```python
from build123d import *

# Parameters (mm, degrees)
F0_R     = 4.7625
F1_DEPTH = 19.05
F4_R     = 6.0191962191


with BuildPart() as f1:
    # F0 (on Top) → F1 (new body)
    with BuildSketch(Plane.XY):
        Polygon((5.2232627241, 4.1654130256), (0, 6.6808037809), (-5.2232627241, 4.1654130256), (-6.5133020818, -1.4866186969), (-2.8986921248, -6.0191962191), (2.8986921248, -6.0191962191), (6.5133020818, -1.4866186969), align=None)
        Circle(F0_R, mode=Mode.SUBTRACT)
        Circle(F0_R)
    extrude(amount=F1_DEPTH)

    # F2 (on face) → F5 section 0
    with BuildSketch(Plane.XY.offset(19.05)):
        with BuildLine():
            ThreePointArc((4.7059970769, -3.7529074911), (5.6814189661, -1.9880145009), (6.0191962191, 0))
            ThreePointArc((6.0191962191, 0), (5.9813487804, 0.6739361184), (5.8682824176, 1.3393970999))
            ThreePointArc((5.8682824176, 1.3393970999), (4.7059971119, 3.7529074472), (2.6116313274, 5.4231084199))
            ThreePointArc((2.6116313274, 5.4231084199), (-1.32e-08, 6.0191962191), (-2.6116313513, 5.4231084084))
            ThreePointArc((-2.6116313513, 5.4231084084), (-4.7059970812, 3.7529074856), (-5.8682823899, 1.3393972216))
            ThreePointArc((-5.8682823899, 1.3393972216), (-5.8682824076, -1.3393971439), (-4.7059970929, -3.752907471))
            ThreePointArc((-4.7059970929, -3.752907471), (-2.6116313545, -5.4231084068), (0, -6.0191962191))
            ThreePointArc((0, -6.0191962191), (2.611631343, -5.4231084124), (4.7059970769, -3.7529074911))
        make_face()
    # F4 (on offset) → F5 section 1
    with BuildSketch(Plane.XY.offset(25.4)):
        Circle(F4_R)
    loft()


solid = f1.part
```
Verification items for the finished model (mm, model axes). A direction names the side the tool comes from. Give positions to 0.01 mm unless a question says otherwise; leave off trailing zeros. Order: outer loops, then holes, each group sorted by start corner. A loop starts at its lowest first (then second) coordinate and runs counter-clockwise, first axis right, second up. Notation, with made-up numbers: (76.25, -36.75) -> (102.25, -36.75) arc R34 cw to (102.25, -6.75) -> close; hole circle Ø7 at (44, -10). An arc over 180 degrees is marked (long way). Use a Markdown table: item, result.
1) Section check B-B, the plane x = -4.25. Record the boundary of the cut face in (y, z).
Results:
| item | result |
|---|---|
| outline | (-4.32, 0) -> (4.63, 0) -> (4.63, 19.05) -> (4.26, 19.05) -> (4.26, 25.4) -> (-4.26, 25.4) -> (-4.26, 19.05) -> (-4.32, 19.05) -> close |
2) Material ranges on probe 1 along X at (y, z) = (3, 20.5); probe 2 along X at (y, z) = (-2.5, 23); probe 3 along Y at (x, z) = (-5, 16.75), recorded low to high.
Results:
| item | result |
|---|---|
| probe 1 | -5.22 to 5.22 |
| probe 2 | -5.48 to 5.48 |
| probe 3 | -3.38 to 4.27 |
3) Depth check by flat-ended pin: pin 1 Ø1.8 at (x, y) = (-3.5, -5) entering from +Z; pin 2 Ø1.5 at (x, z) = (4, 20) entering from -Y; pin 3 Ø5 at (y, z) = (4.5, 9.5) entering from -X; pin 4 Ø3 at (y, z) = (-4.5, 10.5) entering from -X. Enter the tip coordinate at first touch or a pass-through.
Results:
| item | result |
|---|---|
| pin 1 | z = 25.4 |
| pin 2 | y = -5.07 |
| pin 3 | x = -5.72 |
| pin 4 | x = -5.31 |
4) Tool access check on faces 1 (the flat face through (2.7, -5.6, 19.05)), 2 (the flat face through (0, 6.2, 19.05)), 3 (the flat face through (5, 4, 19.05)). Record the directions out of +Z, -Z, +X, -X, +Y, -Y that give a thin tool (end or side, any length) a straight path to the whole face; none if there is none.
Results:
| item | result |
|---|---|
| face 1 | +Z, +X, -Y |
| face 2 | +Z, +Y |
| face 3 | +Z, +X, +Y |
5) Section check A-A, the plane z = 10.5. Record the boundary of the cut face in (x, y), then the cut area to 3 significant figures.
Results:
| item | result |
|---|---|
| outline | (-6.51, -1.49) -> (-2.9, -6.02) -> (2.9, -6.02) -> (6.51, -1.49) -> (5.22, 4.17) -> (0, 6.68) -> (-5.22, 4.17) -> close |
| area | 122 mm² |
